Autodesk Fusion 360 part; units mm, degrees
sketch "Sketch1" plane through (0, 0, 0) normal (0, 1, 0) x (1, 0, 0)
  line L0 (0, 0) -> (41, 0)
  line L1 (41, 0) -> (41, -41)
  line L2 (41, -41) -> (0, -41)
  line L3 (0, -41) -> (0, 0)
  line L4 (0, -20.5) -> (41, -20.5) construction
  line L5 (20.5, 0) -> (20.5, -41) construction
  circle A0 centre (20.5, -20.5) radius 12.5
  line L6 (36, -36) -> (5, -36) construction
  line L7 (5, -36) -> (5, -5) construction
  line L8 (5, -5) -> (36, -5) construction
  line L9 (36, -5) -> (36, -36) construction
  line L10 (36, -36) -> (5, -5) construction
  line L11 (5, -36) -> (36, -5) construction
  circle A1 centre (5, -36) radius 1.8
  circle A2 centre (36, -36) radius 1.8
  circle A3 centre (36, -5) radius 1.8
  circle A4 centre (5, -5) radius 1.8
  circle A5 centre (5, -36) radius 3.25
  circle A6 centre (36, -36) radius 3.25
  circle A7 centre (36, -5) radius 3.25
  circle A8 centre (5, -5) radius 3.25
  line L12 (0, -10.5) -> (13, -10.5)
  line L13 (13, -30.5) -> (0, -30.5)
  point P0 (20.5, -20.5)
  dimension "d1" = 31
  dimension "d2" = 31
  dimension "d3" = 25
  dimension "d4" = 3.6
  dimension "d5" = 3.6
  dimension "d6" = 3.6
  dimension "d7" = 3.6
  dimension "d8" = 6.5
  dimension "d9" = 6.5
  dimension "d10" = 6.5
  dimension "d11" = 6.5
  dimension "d12" = 41
  dimension "d13" = 10
  dimension "d14" = 10
extrude "Extrude1" add sketch "Sketch1" along normal blind 2 contours L0 L1 L2 L3 A0 L12 L13 | A5 | A6 | A7 | A8
extrude "Extrude2" add sketch "Sketch1" along normal blind 22 contours A5 | A6 | A7 | A8
ref_plane "WorkPlane1" through (20.5, 1, 20.5) normal (0, 0, 1) x (1, 0, 0)
fillet "Fillet1" radius 1 4 edges at (32.9699, 2, 34.8247) (32.9699, 2, 3.8247) (1.9699, 2, 3.8247) (1.9699, 2, 34.8247)
fillet "Fillet2" radius 4.5 6 edges at (41, 1, 0) (41, 1, 41) (0, 1, 0) (0, 1, 41) (0, 1, 10.5) (0, 1, 30.5)
equation "d2 = d1"
equation "d5 = d4"
equation "d6 = d5"
equation "d7 = d4"
equation "d9 = d8"
equation "d10 = d8"
equation "d11 = d8"
equation "d14 = d13"
equation "Hoogte = 22 mm"
equation "d18 = Hoogte"
equation "d20 = ( -41 / 2 ) * 1 mm"
The listing builds one solid part. Answer for the finished solid, in the listing's coordinates (mm). A direction names the side the tool comes from. Coordinates: 2 decimals unless noted, no trailing zeros. Write each loop counter-clockwise with the first axis right and the second up, starting at its lowest first coordinate (ties: lowest second). Pieces come first, ordered by that corner, then holes. Notation, with made-up numbers: (-4.75, -8.5) - (48.25, -8.5) arc R26 cw to (48.25, 20.5) - close; hole circle Ø6 at (-9, -17). An arc over 180 degrees is marked (long way). Put each result on its own line as item: value.
1. The part is cut by section B-B on x = 5. Give the vertices of the cut face in (y, z), plus the area to 3 significant figures.
Answer sheet:
outline: (0, 0) - (2, 0) - (2, 0.75) arc R1 cw to (3, 1.75) - (22, 1.75) - (22, 3.2) - (0, 3.2) - close; (0, 6.8) - (22, 6.8) - (22, 8.25) - (3, 8.25) arc R1 cw to (2, 9.25) - (2, 10.5) - (0, 10.5) - close; (0, 30.5) - (2, 30.5) - (2, 31.75) arc R1 cw to (3, 32.75) - (22, 32.75) - (22, 34.2) - (0, 34.2) - close; (0, 37.8) - (22, 37.8) - (22, 39.25) - (3, 39.25) arc R1 cw to (2, 40.25) - (2, 41) - (0, 41) - close
area: 144 mm^2
2. The part is cut by section D-D on x = 36. Give the vertices of the cut face in (y, z).
Answer sheet:
outline: (0, 0) - (2, 0) - (2, 0.75) arc R1 cw to (3, 1.75) - (22, 1.75) - (22, 3.2) - (0, 3.2) - close; (0, 6.8) - (22, 6.8) - (22, 8.25) - (3, 8.25) arc R1 cw to (2, 9.25) - (2, 31.75) arc R1 cw to (3, 32.75) - (22, 32.75) - (22, 34.2) - (0, 34.2) - close; (0, 37.8) - (22, 37.8) - (22, 39.25) - (3, 39.25) arc R1 cw to (2, 40.25) - (2, 41) - (0, 41) - close
3. Determine the mould class of faces 4 (the face through (9, 1, 10.5)), 5 (the face through (34, 0, 20)), 6 (the face through (39.647, 1.014, 39.717)) for opening direction Z: pulls with the +Z half, pulls with the -Z half, needs draft (parallel to the pull), parting line crosses it, or undercut.
Answer sheet:
face 4: undercut
face 5: needs draft
face 6: pulls with the +Z half
4. Find the intervals of material crossed by line 1 along Z through (x, y) = (5, 5.5); line 2 along Z through (x, y) = (35, 7.75), in increasing order. Write a range as from..to.
Answer sheet:
line 1: z = 1.75..3.2, 6.8..8.25, 32.75..34.2, 37.8..39.25
line 2: z = 1.91..3.5, 6.5..8.09, 32.91..34.5, 37.5..39.09
5. The part is cut by section C-C on x = 20.5. Give the vertices of the cut face in (y, z).
Answer sheet:
outline: (0, 0) - (2, 0) - (2, 8) - (0, 8) - close; (0, 33) - (2, 33) - (2, 41) - (0, 41) - close
6. Flat-ended cylindrical pins translate along their axes: pin 1 Ø8 at (x, y) = (8.5, 9.5) entering from -Z; pin 2 Ø6 at (x, z) = (29.5, 27) entering from +Y; pin 3 Ø6 at (x, z) = (36, 36) entering from +Y. Find the tip coordinate at first contact, or state that the pin passes through.
Answer sheet:
pin 1: stops at z = 1.75
pin 2: stops at y = 2
pin 3: stops at y = 22
7. The part is cut by section A-A on y = 12. Give the vertices of the cut face in (x, z), plus the area to 3 significant figures.
Answer sheet:
outline: circle Ø6.5 at (5, 5); circle Ø6.5 at (5, 36); circle Ø6.5 at (36, 5); circle Ø6.5 at (36, 36); hole circle Ø3.6 at (5, 5); hole circle Ø3.6 at (5, 36); hole circle Ø3.6 at (36, 5); hole circle Ø3.6 at (36, 36)
area: 92.0 mm^2
8. A tool of negligible diameter and unlimited length cuts with its end or side. For faces 1 (the face through (1.283, 1.014, 9.147)), 2 (the face through (39.717, 1.014, 1.353)), 3 (the face through (8.1, 12.37, 5.98)), from which of +Z, -Z, +X, -X, +Y, -Y can it reach the whole face along a straight path? Write none if from no direction.
Answer sheet:
face 1: -X, +Y, -Y
face 2: -Z, +X, +Y, -Y
face 3: +Y
